Autodesk Inventor part; units mm, degrees
ref_plane "YZ Plane" through (0, 0, 0) normal (1, 0, 0) x (0, 1, 0)
ref_plane "XZ Plane" through (0, 0, 0) normal (0, 1, 0) x (-1, 0, 0)
ref_plane "XY Plane" through (0, 0, 0) normal (0, 0, 1) x (1, 0, 0)
sketch "Sketch1" plane through (0, 0, 0) normal (0, 0, 1) x (1, 0, 0)
  circle A0 centre (0, 0) radius 10
  circle A1 centre (0, 0) radius 4
  point P0 (-10, 0)
  dimension "d0" = 20
  dimension "d1" = 8
extrude "Extrusion1" add sketch "Sketch1" along normal mid plane 25.2 contours A1
extrude "Extrusion2" add sketch "Sketch1" along normal mid plane 20
hole "Hole1" at (-10, 0, 0) direction (1, 0, 0) diameter 8.376 end through all
chamfer "Chamfer1" distance 1 angle 45 8 edges at (9.4815, 3.1784, 2.7271) (9.4815, -3.1783, 2.7272) (9.4815, -3.1784, -2.7271) (9.4815, 3.1783, -2.7272) (-9.4815, 3.1784, 2.7271) (-9.4815, 3.1783, -2.7272) (-9.4815, -3.1784, -2.7271) (-9.4815, -3.1783, 2.7272)
properties part number "BaseSpacer" material "Steel, Mild"
The listing builds one solid part. Answer for the finished solid, in the listing's coordinates (mm). A direction names the side the tool comes from. Round coordinates to 2 decimals unless told otherwise and drop trailing zeros. Write each loop counter-clockwise with the first axis right and the second up, starting at its lowest first coordinate (ties: lowest second). Pieces come first, ordered by that corner, then holes. Notation, with made-up numbers: (4, -26) - (28, -26) arc R35 ccw to (28, 9) - close; hole circle Ø8 at (-37.75, -20.75). An arc over 180 degrees is marked (long way). Use a Markdown table: item, result. Add a question column.
1. The part is cut by section A-A (x = 0). Write down the section's boundary in (y, z).
2. The part is cut by section C-C (y = -7.25). Write down the section's boundary in (x, z), and give its area (4 significant figures).
3. A tool of negligible diameter and unlimited length cuts with its end or side. For faces 4 (the face through (-0.867, 3.905, 11.282)), 5 (the face through (0, 0, -12.6)), 6 (the face through (-0.867, -3.905, -11.282)), from which of +Z, -Z, +X, -X, +Y, -Y can it reach the whole face along a straight path? Write none if from no direction.
4. For a pull along Y with two mould halves and no side action, classify faces 1 (the face through (0.125, -1.258, 3.995)), 2 (the face through (-8, 6, 0)), 3 (the face through (4.3, 0.1, 10)) as +Y half, -Y half, draft (parallel to the pull), parting line (faces both ways), or undercut.
5. Flat-ended cylindrical pins translate along their axes: P1, Ø5, axis at x = 3.5, z = 5, coming from the +Y side; P2, Ø3, axis at y = 3, z = -4.5, coming from the -X side; P3, Ø8, axis at y = 8, z = -5.5, coming from the +X side; P4, Ø5, axis at y = 0, z = 0, coming from the +X side. Find the tip coordinate at first contact, or state that the pin passes through.
6. Consider line 1 (Z direction, x = 3.5, y = 0); line 2 (Y direction, x = -4, z = 0); line 3 (Y direction, x = 2, z = 0). Determine where each line is inside the solid, lowest interval first.
7. The part is cut by section B-B (z = 11). Write down the section's boundary in (x, y), and give its area (3 significant figures).
8. The part is cut by section D-D (x = -6.25). Write down the section's boundary in (y, z), and give its area (3 significant figures).
Reported:
| question | item | result |
|---|---|---|
| 1 | outline | (-10, -10) - (-4, -10) - (-4, -12.6) - (4, -12.6) - (4, -10) - (10, -10) - (10, 10) - (4, 10) - (4, 12.6) - (-4, 12.6) - (-4, 10) - (-10, 10) - close; hole circle Ø8.38 at (0, 0) |
| 2 | outline | (-6.89, -10) - (6.89, -10) - (6.89, 10) - (-6.89, 10) - close |
| 2 | area | 275.5 mm^2 |
| 3 | face 4 | +Z |
| 3 | face 5 | -Z, +X, -X, +Y, -Y |
| 3 | face 6 | -Z |
| 4 | face 1 | undercut |
| 4 | face 2 | parting line |
| 4 | face 3 | draft |
| 5 | P1 | y = 9.95 |
| 5 | P2 | x = -9.88 |
| 5 | P3 | x = 9.17 |
| 5 | P4 | through |
| 6 | line 1 | -12.6 to -4.19, 4.19 to 12.6 |
| 6 | line 2 | -9.17 to -4.19, 4.19 to 9.17 |
| 6 | line 3 | -9.8 to -4.19, 4.19 to 9.8 |
| 7 | outline | circle Ø8 at (0, 0) |
| 7 | area | 50.3 mm^2 |
| 8 | outline | (-7.81, -10) - (7.81, -10) - (7.81, 10) - (-7.81, 10) - close; hole circle Ø8.38 at (0, 0) |
| 8 | area | 257 mm^2 |
